Read the model definition and answer for the solid it produces. Units are mm, in the model's axes. Coordinates: 2 decimals unless noted, no trailing zeros. Order: outer loops, then holes, each group sorted by start corner. A loop starts at its lowest first (then second) coordinate and runs counter-clockwise, first axis right, second up. Notation, with made-up numbers: M 40.5,-19.75 L 68.5,-19.75 A12 ccw 68.5,-0.75 Z; hole C -25,-36.75 d9. An arc over 180 degrees is marked long. Use a Markdown table: item, result. Add a question column.
1) Each of these flat-tipped pins is pushed along its axis until it touches: pin 1 Ø2.5 at (x, z) = (-71, -1) entering from +Y; pin 2 Ø1 at (y, z) = (-34.5, -1.5) entering from +X; pin 3 Ø1.5 at (y, z) = (44.5, 1.5) entering from -X. Where does it stop, or does it pass through?
2) Find section C-C on y = 39. Write down the section's boundary in (x, z), plus the area to 3 significant figures.
3) Find section A-A on z = 1.25. Write down the section's boundary in (x, y), plus the area to 3 significant figures.
4) Find section B-B on x = -82. Write down the section's boundary in (y, z).
5) Find the intervals of material crossed by probe 1 along X at (y, z) = (95.5, 1.5); probe 2 along X at (y, z) = (-99, 0.65); probe 3 along Y at (x, z) = (-141, 1.6), in increasing order. Write a range as [from, to].
from build123d import *

# Parameters (mm, degrees)
BOSS_EXTRUDE1_DEPTH = 2.5


with BuildPart() as part:
    # Sketch1 → Boss-Extrude1 (new, symmetric)
    with BuildSketch(Plane.XY):
        Polygon((163.713404947, -144.224375), (163.713404947, -118.030625), (20.889204947, 118.030625), (-150.230595053, 118.030625), (-150.230595053, 127.022225), (-169.153595053, 127.022225), (-65.280574469, -44.660130514), (19.852041127, -74.374375), (62.113404947, -144.224375), align=None)
    extrude(amount=BOSS_EXTRUDE1_DEPTH, both=True)


solid = part.part
Check result:
| question | item | result |
|---|---|---|
| 1 | pin 1 | stops at y = 118.03 |
| 1 | pin 2 | stops at x = 113.48 |
| 1 | pin 3 | stops at x = -119.68 |
| 2 | outline | M -115.9,-2.5 L 68.71,-2.5 L 68.71,2.5 L -115.9,2.5 Z |
| 2 | area | 923 mm2 |
| 3 | outline | M -169.15,127.02 L -65.28,-44.66 L 19.85,-74.37 L 62.11,-144.22 L 163.71,-144.22 L 163.71,-118.03 L 20.89,118.03 L -150.23,118.03 L -150.23,127.02 Z |
| 3 | area | 42,700 mm2 |
| 4 | outline | M -17.03,-2.5 L 118.03,-2.5 L 118.03,2.5 L -17.03,2.5 Z |
| 5 | probe 1 | x = [-150.08, 34.52] |
| 5 | probe 2 | x = [34.75, 152.2] |
| 5 | probe 3 | y = [80.49, 118.03] |
